```python
from build123d import *

# Parameters (mm, degrees)
ESQUISSE1_W             = 60
ESQUISSE1_H             = 16.26
ESQUISSE1_R             = 8
BOSS_EXTRU_1_DEPTH      = 9
ESQUISSE2_W             = 11
ESQUISSE2_H             = 4
BOSS_EXTRU_2_DEPTH      = 9
ESQUISSE3_W             = 12
ESQUISSE3_H             = 3
BOSS_EXTRU_3_DEPTH      = 9
CHANFREIN2_SIZE         = 3
ESQUISSE4_R             = 2
ENL_V_MAT_EXTRU_1_DEPTH = 64.964580824


with BuildPart() as part:
    # Esquisse1 → Boss.-Extru.1 (new body)
    with BuildSketch(Plane.XY):
        with Locations((30, 8.13)):
            Rectangle(ESQUISSE1_W, ESQUISSE1_H)
        with Locations((30, 8.13)):
            Circle(ESQUISSE1_R, mode=Mode.SUBTRACT)
    extrude(amount=BOSS_EXTRU_1_DEPTH)

    # Esquisse2 → Boss.-Extru.2 (add)
    with BuildSketch(Plane.XY.offset(9)):
        with Locations((30, 18.26)):
            Rectangle(ESQUISSE2_W, ESQUISSE2_H)
    extrude(amount=-BOSS_EXTRU_2_DEPTH)

    # Esquisse3 → Boss.-Extru.3 (add)
    with BuildSketch(Plane.XY.offset(9)):
        with Locations((30, -1.5)):
            Rectangle(ESQUISSE3_W, ESQUISSE3_H)
    extrude(amount=-BOSS_EXTRU_3_DEPTH)

    # Chanfrein2
    chanfrein2_edges = [part.edges().sort_by_distance(p)[0] for p in [
        (36, 0, 4.5),
        (24, 0, 4.5),
    ]]
    chamfer(chanfrein2_edges, length=CHANFREIN2_SIZE - 0.0001)  # a hair under: the kernel refuses the full size

    # Esquisse4 → Enlèv. mat.-Extru.1 (cut, through all)
    with BuildSketch(Plane.XZ):
        with Locations(Location((17, 4.5, 0), (0, 0, 270))):
            Circle(ESQUISSE4_R)
        with Locations(Location((5, 4.5, 0), (0, 0, 270))):
            Circle(ESQUISSE4_R)
        with Locations(Location((55, 4.5, 0), (0, 0, 270))):
            Circle(ESQUISSE4_R)
        with Locations(Location((43, 4.5, 0), (0, 0, 270))):
            Circle(ESQUISSE4_R)
    extrude(amount=-ENL_V_MAT_EXTRU_1_DEPTH, mode=Mode.SUBTRACT)


solid = part.part
```
Check sheet for the modelled part. Datum: model origin and axes. Units: mm. A direction names the side the tool comes from. Give positions to 0.01 mm unless a question says otherwise; leave off trailing zeros. Write each loop counter-clockwise with the first axis right and the second up, starting at its lowest first coordinate (ties: lowest second). Pieces come first, ordered by that corner, then holes. Notation, with made-up numbers: (74, 50) -> (85, 50) arc R13 cw to (85, 70) -> close; hole circle Ø4 at (74, -11). An arc over 180 degrees is marked (long way). Use CSV: the item, a comma, the result in double quotes. Start each with the question number.
Q1. Cross-section at A-A on y = 8.13. Enter the section's corners in (x, z).
Q2. Cross-section at B-B on z = 4.5. Count the separate pieces of the cut face and the enclosed holes in it, and give its area (3 significant figures).
Q3. Scan lines: line 1 along X through (y, z) = (7.75, 4.5); line 2 along Y through (x, z) = (30, 5.5); line 3 along X through (y, z) = (11.75, 4.5). Record each from-to range of solid material in increasing order.
Q4. Tool access check on faces 4 (the flat face through (10, 0, 4)), 5 (the flat face through (49, 0, 4)), 6 (the flat face through (35.5, 18, 5)). Record the directions out of +Z, -Z, +X, -X, +Y, -Y that give a thin tool (end or side, any length) a straight path to the whole face; none if there is none.
Q5. Release check for a two-part mould opening along Z. For faces 1 (the flat face through (22.9, 3.6, 0)), 2 (the cylindrical face through (41.048, 8.016, 4.934)), 3 (the flat face through (30, -3, 5)) record: +Z half, -Z half, draft (parallel to the pull), parting line (faces both ways), or undercut.
Q6. Depth check by flat-ended pin: P1, Ø4.5, axis at x = 55, z = 4.5, coming from the -Y side; P2, Ø8, axis at x = 47.5, y = 17, coming from the -Z side; P3, Ø2, axis at y = 19, z = 4.5, coming from the -X side; P4, Ø4.5, axis at x = 17.5, z = 5, coming from the +Y side. Enter the tip coordinate at first touch or a pass-through.
Q7. Cross-section at C-C on x = 17. Enter the section's corners in (y, z).
Working result:
1,outline,"(0, 0) -> (22, 0) -> (22, 9) -> (0, 9) -> close; (38, 0) -> (60, 0) -> (60, 9) -> (38, 9) -> close; hole circle Ø4 at (5, 4.5); hole circle Ø4 at (17, 4.5); hole circle Ø4 at (43, 4.5); hole circle Ø4 at (55, 4.5)"
2,separate pieces,"5"
2,enclosed holes,"1"
2,area,"603 mm^2"
3,line 1,"x = 0 to 3, 7 to 15, 19 to 22.01, 37.99 to 41, 45 to 53, 57 to 60"
3,line 2,"y = -3 to 0.13, 16.13 to 20.26"
3,line 3,"x = 0 to 3, 7 to 15, 19 to 22.87, 37.13 to 41, 45 to 53, 57 to 60"
4,face 4,"+Z, -Z, -X, -Y"
4,face 5,"+Z, -Z, +X, -Y"
4,face 6,"+Z, -Z, +X, +Y"
5,face 1,"-Z half"
5,face 2,"undercut"
5,face 3,"draft"
6,P1,"stops at y = 0"
6,P2,"stops at z = 0"
6,P3,"stops at x = 24.5"
6,P4,"stops at y = 16.26"
7,outline,"(0, 0) -> (16.26, 0) -> (16.26, 2.5) -> (0, 2.5) -> close; (0, 6.5) -> (16.26, 6.5) -> (16.26, 9) -> (0, 9) -> close"
